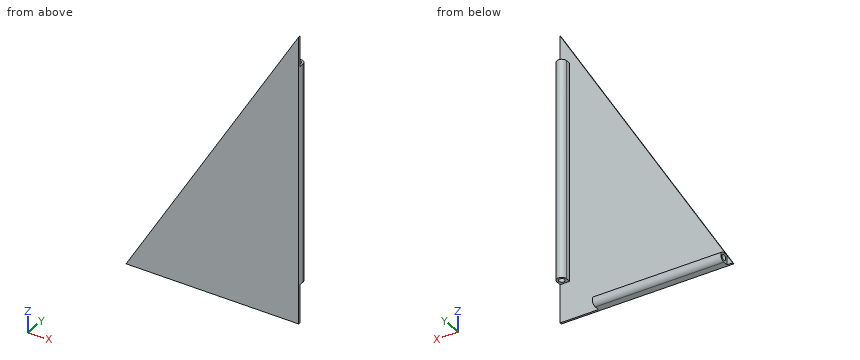
Autodesk Fusion 360 part; units mm, degrees
sketch "スケッチ1" plane through (0, 0, 0) normal (0, 1, 0) x (1, 0, 0)
  line L0 (0, 0) -> (0, -150)
  line L1 (0, 0) -> (-90, 0)
  line L2 (-90, 0) -> (0, -150)
  dimension "d1" = 150
  dimension "d2" = 90
extrude "押し出し1" add sketch "スケッチ1" along normal blind 1
ref_plane "作業平面1" through (-45, 0.5, 20) normal (0, 0, -1) x (-1, 0, 0)
sketch "スケッチ2" plane through (0, 0, 20) normal (0, 0, -1) x (-1, 0, 0)
  circle A0 centre (2.5, 3.5) radius 1.5
  line L0 (0, 1) -> (90, 1)
  line L1 (0, 1.75) -> (0, 22.5)
  circle A1 centre (2.5, 3.5) radius 2.5
  line L2 (5, 3.5) -> (5, 1)
  line L3 (0, 3.5) -> (0, 1)
  dimension "d6" = 3
  dimension "d7" = 1
extrude "押し出し2" add sketch "スケッチ2" against normal blind 114
ref_plane "作業平面2" through (-20, 1.75, 75) normal (1, 0, 0) x (0, 0, -1)
sketch "スケッチ3" plane through (-20, 0, 0) normal (1, 0, 0) x (0, 0, -1)
  circle A0 centre (-2.5, 3.5) radius 1.5
  circle A1 centre (-2.5, 3.5) radius 2.5
  line L0 (-20, 1) -> (0, 1)
  line L1 (0, 1.75) -> (0, 22.5)
  line L2 (0, 3.5) -> (0, 1)
  line L3 (-5, 3.5) -> (-5, 1)
  dimension "d11" = 3
  dimension "d12" = 1
extrude "押し出し3" add sketch "スケッチ3" against normal blind 67
Read the model definition and answer for the solid it produces. Units are mm, in the model's axes. Give positions to 0.01 mm unless a question says otherwise; leave off trailing zeros. Write each loop counter-clockwise with the first axis right and the second up, starting at its lowest first coordinate (ties: lowest second). Pieces come first, ordered by that corner, then holes. Notation, with made-up numbers: (50.25, -4.5) -> (82.25, -4.5) arc R18 ccw to (82.25, 24.5) -> close; hole circle Ø11 at (16, 37.5). An arc over 180 degrees is marked (long way). Answer in a Markdown table with one row per item.
1) Each of these flat-tipped pins is pushed along its axis until it touches: pin 1 Ø6 at (x, z) = (-10.5, 132.5) entering from +Y; pin 2 Ø2.5 at (y, z) = (4, 3) entering from -X; pin 3 Ø1.5 at (x, y) = (-1.5, 3.5) entering from +Z; pin 4 Ø2.5 at (y, z) = (3.5, 2.5) entering from -X. Where does it stop, or does it pass through?
Results list:
| item | result |
|---|---|
| pin 1 | y = 1 |
| pin 2 | x = -87 |
| pin 3 | z = 134 |
| pin 4 | through |
2) Section C-C on x = -2.5 is taken. Give the vertices of the cut face in (y, z), plus the area to 3 significant figures.
Results list:
| item | result |
|---|---|
| outline | (0, 0) -> (1, 0) -> (1, 20) -> (2, 20) -> (2, 134) -> (1, 134) -> (1, 145.83) -> (0, 145.83) -> close; (5, 20) -> (6, 20) -> (6, 134) -> (5, 134) -> close |
| area | 374 mm^2 |
3) Section B-B on x = -81 is taken. Give the vertices of the cut face in (y, z).
Results list:
| item | result |
|---|---|
| outline | (0, 0) -> (3.5, 0) arc R2.5 ccw to (3.5, 5) -> (1, 5) -> (1, 15) -> (0, 15) -> close; hole circle Ø3 at (3.5, 2.5) |
4) Straight lines are drawn through the part: line 1 (Y direction, x = -66, z = 2.5); line 2 (X direction, y = 3.7, z = 106); line 3 (Z direction, x = -4.5, y = 2.95). For each, find the intervals that lie inside material, in ascending order. Write a range as [from, to].
Results list:
| item | result |
|---|---|
| line 1 | [0, 2], [5, 6] |
| line 2 | [-4.99, -3.99], [-1.01, -0.01] |
| line 3 | [20, 134] |
5) Section D-D on z = 24 is taken. Give the vertices of the cut face in (x, y), plus the area to 3 significant figures.
Results list:
| item | result |
|---|---|
| outline | (-75.6, 0) -> (0, 0) -> (0, 3.5) arc R2.5 ccw to (-5, 3.5) -> (-5, 1) -> (-75.6, 1) -> close; hole circle Ø3 at (-2.5, 3.5) |
| area | 90.8 mm^2 |
6) Section A-A on z = 2.5 is taken. Give the vertices of the cut face in (x, y).
Results list:
| item | result |
|---|---|
| outline | (-88.5, 0) -> (0, 0) -> (0, 1) -> (-20, 1) -> (-20, 2) -> (-87, 2) -> (-87, 1) -> (-88.5, 1) -> close; (-87, 5) -> (-20, 5) -> (-20, 6) -> (-87, 6) -> close |
